Read the model definition and answer for the solid it produces. Units are mm, in the model's axes. A direction names the side the tool comes from. Coordinates: 2 decimals unless noted, no trailing zeros. Write each loop counter-clockwise with the first axis right and the second up, starting at its lowest first coordinate (ties: lowest second). Pieces come first, ordered by that corner, then holes. Notation, with made-up numbers: (61.25, 40.25) -> (109.25, 40.25) arc R31 cw to (109.25, 71.25) -> close; hole circle Ø9 at (-30, -31.5). An arc over 180 degrees is marked (long way). Return JSON: item names as keys, results as strings.
from build123d import *

# Parameters (mm, degrees)
SKETCH1_W           = 250
SKETCH1_H           = 350
BOSS_EXTRUDE1_DEPTH = 7
SKETCH2_W           = 14
SKETCH2_H           = 42
CUT_EXTRUDE1_DEPTH  = 281.478441071
SKETCH3_W           = 14
SKETCH3_H           = 42
CUT_EXTRUDE2_DEPTH  = 281.478441071
SKETCH4_W           = 74
SKETCH4_H           = 12
CUT_EXTRUDE3_DEPTH  = 281.478441071
SKETCH5_W           = 54
SKETCH5_H           = 22
CUT_EXTRUDE4_DEPTH  = 281.478441071
SKETCH6_R           = 11
CUT_EXTRUDE5_DEPTH  = 281.478441071


with BuildPart() as part:
    # Sketch1 → Boss-Extrude1 (new body)
    with BuildSketch(Plane(origin=(0, 0, 0), x_dir=(1, 0, 0), z_dir=(0, 1, 0))):
        with Locations((2.912621359, -74.514563107)):
            Rectangle(SKETCH1_W, SKETCH1_H)
    extrude(amount=BOSS_EXTRUDE1_DEPTH)

    # Sketch2 → Cut-Extrude1 (cut, through all)
    with BuildSketch(Plane(origin=(0, 7, 0), x_dir=(1, 0, 0), z_dir=(0, 1, 0))):
        with Locations((-104.087378641, 46.485436893)):
            Rectangle(SKETCH2_W, SKETCH2_H)
        with Locations((-74.087378641, 46.485436893)):
            Rectangle(SKETCH2_W, SKETCH2_H)
        with Locations((-44.087378641, 46.485436893)):
            Rectangle(SKETCH2_W, SKETCH2_H)
        with Locations((-14.087378641, 46.485436893)):
            Rectangle(SKETCH2_W, SKETCH2_H)
        with Locations((15.912621359, 46.485436893)):
            Rectangle(SKETCH2_W, SKETCH2_H)
        with Locations((45.912621359, 46.485436893)):
            Rectangle(SKETCH2_W, SKETCH2_H)
        with Locations((75.912621359, 46.485436893)):
            Rectangle(SKETCH2_W, SKETCH2_H)
        with Locations((105.912621359, 46.485436893)):
            Rectangle(SKETCH2_W, SKETCH2_H)
    extrude(amount=-CUT_EXTRUDE1_DEPTH, mode=Mode.SUBTRACT)

    # Sketch3 → Cut-Extrude2 (cut, through all)
    with BuildSketch(Plane(origin=(0, 7, 0), x_dir=(1, 0, 0), z_dir=(0, 1, 0))):
        with Locations((-92.087378641, -132.514563107)):
            Rectangle(SKETCH3_W, SKETCH3_H)
        with Locations((-62.087378641, -132.514563107)):
            Rectangle(SKETCH3_W, SKETCH3_H)
    extrude(amount=-CUT_EXTRUDE2_DEPTH, mode=Mode.SUBTRACT)

    # Sketch4 → Cut-Extrude3 (cut, through all)
    with BuildSketch(Plane(origin=(0, 7, 0), x_dir=(1, 0, 0), z_dir=(0, 1, 0))):
        with Locations((-71.087378641, -34.514563107)):
            Rectangle(SKETCH4_W, SKETCH4_H)
    extrude(amount=-CUT_EXTRUDE3_DEPTH, mode=Mode.SUBTRACT)

    # Sketch5 → Cut-Extrude4 (cut, through all)
    with BuildSketch(Plane(origin=(0, 7, 0), x_dir=(1, 0, 0), z_dir=(0, 1, 0))):
        with Locations((80.912621359, -138.514563107)):
            Rectangle(SKETCH5_W, SKETCH5_H)
    extrude(amount=-CUT_EXTRUDE4_DEPTH, mode=Mode.SUBTRACT)

    # Sketch6 → Cut-Extrude5 (cut, through all)
    with BuildSketch(Plane(origin=(0, 7, 0), x_dir=(1, 0, 0), z_dir=(0, 1, 0))):
        with Locations(Location((100.912621359, -48.514563107, 0), (0, 0, 270))):
            Circle(SKETCH6_R)
        with Locations(Location((68.333659496, -48.514563107, 0), (0, 0, 270))):
            Circle(SKETCH6_R)
    extrude(amount=-CUT_EXTRUDE5_DEPTH, mode=Mode.SUBTRACT)


solid = part.part
1. For a pull along X with two mould halves and no side action, classify faces 1 (the face through (1, 3, 249.515)), 2 (the face through (-122.087, 3, 77)), 3 (the face through (-69.087, 4, 133)) as +X half, -X half, draft (parallel to the pull), parting line (faces both ways), or undercut.
Taken from the geometry:
{"face 1": "draft", "face 2": "-X half", "face 3": "undercut"}
2. The part is cut by section A-A (x = -59.5). Determine the outline of the cut face in (y, z), then the cut area to 3 significant figures.
Taken from the geometry:
{"outline": "(0, -100.49) -> (7, -100.49) -> (7, 28.51) -> (0, 28.51) -> close; (0, 40.51) -> (7, 40.51) -> (7, 111.51) -> (0, 111.51) -> close; (0, 153.51) -> (7, 153.51) -> (7, 249.51) -> (0, 249.51) -> close", "area": "2,070 mm2"}
3. The part is cut by section D-D (y = 3.75). Count the separate pieces of the cut face and the enclosed holes in it, then the cut area to 3 significant figures.
Taken from the geometry:
{"separate pieces": "1", "enclosed holes": "14", "area": "78,800 mm2"}
4. Consider L1, parallel to Z at x = -71, y = 4.75; L2, parallel to Z at x = -86, y = 1; L3, parallel to X at y = 1.5, z = 153. Determine where each line is inside the solid, lowest interval first.
Taken from the geometry:
{"L1": "z = -100.49 to -67.49, -25.49 to 28.51, 40.51 to 249.51", "L2": "z = -100.49 to 28.51, 40.51 to 111.51, 153.51 to 249.51", "L3": "x = -122.09 to -99.09, -85.09 to -69.09, -55.09 to 127.91"}
5. A tool of negligible diameter and unlimited length cuts with its end or side. For faces 4 (the face through (1, 0, 72)), 5 (the face through (-14, 4, -25.485)), from which of +Z, -Z, +X, -X, +Y, -Y can it reach the whole face along a straight path? Write none if from no direction.
Taken from the geometry:
{"face 4": "+Z, -Z, +X, -X, -Y", "face 5": "+Y, -Y"}
6. The part is cut by section B-B (x = 18.5). Determine the outline of the cut face in (y, z), then the cut area to 3 significant figures.
Taken from the geometry:
{"outline": "(0, -100.49) -> (7, -100.49) -> (7, -67.49) -> (0, -67.49) -> close; (0, -25.49) -> (7, -25.49) -> (7, 249.51) -> (0, 249.51) -> close", "area": "2,160 mm2"}
7. The part is cut by section C-C (z = 50). Determine the outline of the cut face in (x, y), then the cut area to 3 significant figures.
Taken from the geometry:
{"outline": "(-122.09, 0) -> (57.43, 0) -> (57.43, 7) -> (-122.09, 7) -> close; (79.23, 0) -> (90.01, 0) -> (90.01, 7) -> (79.23, 7) -> close; (111.81, 0) -> (127.91, 0) -> (127.91, 7) -> (111.81, 7) -> close", "area": "1,440 mm2"}
8. Flat-ended cylindrical pins translate along their axes: pin 1 Ø8 at (x, z) = (76.5, 111) entering from -Y; pin 2 Ø17.5 at (x, z) = (100.91, 48.51) entering from -Y. Find the tip coordinate at first contact, or state that the pin passes through.
Taken from the geometry:
{"pin 1": "stops at y = 0", "pin 2": "passes through"}
